Design review of the part built by this model. Coordinates are the model's own, in mm. A direction names the side the tool comes from. Give positions to 0.01 mm unless a question says otherwise; leave off trailing zeros. Order: outer loops, then holes, each group sorted by start corner. A loop starts at its lowest first (then second) coordinate and runs counter-clockwise, first axis right, second up. Notation, with made-up numbers: M -33,61.5 L 1,61.5 A23 ccw 1,71.5 Z; hole C 9,37 d2. An arc over 180 degrees is marked long. Answer as a JSON object with one key per item and string values.
from build123d import *

# Parameters (mm, degrees)
BOSS_EXTRUDE1_DEPTH = 32
SKETCH4_R           = 16
CUT_EXTRUDE3_DEPTH  = 15
SKETCH5_R           = 7
SKETCH5_R_2         = 4
BOSS_EXTRUDE2_DEPTH = 17
SKETCH15_W          = 16
SKETCH15_H          = 32
CUT_EXTRUDE6_DEPTH  = 15
SKETCH16_W          = 32
SKETCH16_H          = 32
BOSS_EXTRUDE6_DEPTH = 20
SKETCH17_R          = 1.75
CUT_EXTRUDE8_DEPTH  = 49
SKETCH18_R          = 1.75
CUT_EXTRUDE9_DEPTH  = 51.695167423
CUT_EXTRUDE10_START = -10
CUT_EXTRUDE10_DEPTH = 5
SKETCH20_R          = 4.25
CUT_EXTRUDE11_DEPTH = 29


with BuildPart() as part:
    # Sketch1 → Boss-Extrude1 (new body)
    with BuildSketch(Plane(origin=(0, 0, 0), x_dir=(0, -1, 0), z_dir=(1, 0, 0))):
        with BuildLine():
            ThreePointArc((-16, 0), (0, 16), (16, 0))
            Line((16, 0), (16, 25))
            Line((16, 25), (-16, 25))
            Line((-16, 25), (-16, 0))
        make_face()
        with BuildLine():
            ThreePointArc((-4.5, 0), (0, 4.5), (4.5, 0))
            Line((4.5, 0), (16, 0))
            ThreePointArc((16, 0), (0, 16), (-16, 0))
            Line((-16, 0), (-4.5, 0))
        make_face()
        with BuildLine():
            Line((16, 0), (4.5, 0))
            ThreePointArc((4.5, 0), (0, -4.5), (-4.5, 0))
            Line((-4.5, 0), (-16, 0))
            ThreePointArc((-16, 0), (0, -16), (16, 0))
        make_face()
        with BuildLine():
            ThreePointArc((-4.5, 0), (0, 4.5), (4.5, 0))
            Line((4.5, 0), (16, 0))
            ThreePointArc((16, 0), (0, 16), (-16, 0))
            Line((-16, 0), (-4.5, 0))
        make_face()
        with BuildLine():
            Line((16, 0), (4.5, 0))
            ThreePointArc((4.5, 0), (0, -4.5), (-4.5, 0))
            Line((-4.5, 0), (-16, 0))
            ThreePointArc((-16, 0), (0, -16), (16, 0))
        make_face()
    extrude(amount=BOSS_EXTRUDE1_DEPTH)

    # Sketch4 → Cut-Extrude3 (cut)
    with BuildSketch(Plane.ZY):
        Circle(SKETCH4_R)
    extrude(amount=-CUT_EXTRUDE3_DEPTH, mode=Mode.SUBTRACT)

    # Sketch5 → Boss-Extrude2 (add)
    with BuildSketch(Plane.ZY.offset(-15)):
        Circle(SKETCH5_R)
        Circle(SKETCH5_R_2, mode=Mode.SUBTRACT)
    extrude(amount=-BOSS_EXTRUDE2_DEPTH)

    # Sketch15 → Cut-Extrude6 (cut)
    with BuildSketch(Plane.ZY):
        with Locations((-8, 0)):
            Rectangle(SKETCH15_W, SKETCH15_H)
    extrude(amount=-CUT_EXTRUDE6_DEPTH, mode=Mode.SUBTRACT)

    # Sketch16 → Boss-Extrude6 (add)
    with BuildSketch(Plane(origin=(0, 0, -25), x_dir=(-1, 0, 0), z_dir=(0, 0, -1))):
        with Locations((-16, 0)):
            Rectangle(SKETCH16_W, SKETCH16_H)
    extrude(amount=BOSS_EXTRUDE6_DEPTH)

    # Sketch17 → Cut-Extrude8 (cut, through all)
    with BuildSketch(Plane.XY.offset(-16)):
        with Locations((4, 0)):
            Circle(SKETCH17_R)
        with Locations((16, 12)):
            Circle(SKETCH17_R)
        with Locations((28, 0)):
            Circle(SKETCH17_R)
        with Locations((16, -12)):
            Circle(SKETCH17_R)
    extrude(amount=-CUT_EXTRUDE8_DEPTH, mode=Mode.SUBTRACT)

    # Sketch18 → Cut-Extrude9 (cut, through all)
    with BuildSketch(Plane.ZY.offset(-15)):
        with Locations((0, 12)):
            Circle(SKETCH18_R)
        with Locations((0, -12)):
            Circle(SKETCH18_R)
        with Locations((12, 0)):
            Circle(SKETCH18_R)
        with Locations(Location((-12, 0, 0), (0, 0, 180))):
            Circle(SKETCH18_R)
    extrude(amount=-CUT_EXTRUDE9_DEPTH, mode=Mode.SUBTRACT)

    # Sketch19 → Cut-Extrude10 (cut)
    with BuildSketch(Plane(origin=(0, 0, -45), x_dir=(-1, 0, 0), z_dir=(0, 0, -1)).offset(CUT_EXTRUDE10_START)):
        Polygon((0, 3), (-5.732050808, 3), (-7.464101615, 0), (-5.732050808, -3), (0, -3), align=None)
        Polygon((-16, -8.535898385), (-19, -10.267949192), (-19, -16), (-13, -16), (-13, -10.267949192), align=None)
        Polygon((-24.535898385, 0), (-26.267949192, 3), (-32, 3), (-32, -3), (-26.267949192, -3), align=None)
        Polygon((-16, 8.535898385), (-13, 10.267949192), (-13, 16), (-19, 16), (-19, 10.267949192), align=None)
    extrude(amount=-CUT_EXTRUDE10_DEPTH, mode=Mode.SUBTRACT)

    # Sketch20 → Cut-Extrude11 (cut)
    with BuildSketch(Plane(origin=(0, 0, -45), x_dir=(-1, 0, 0), z_dir=(0, 0, -1))):
        with Locations((-16, 0)):
            Circle(SKETCH20_R)
    extrude(amount=-CUT_EXTRUDE11_DEPTH, mode=Mode.SUBTRACT)


solid = part.part
(1) Insertion check: pin 1 (4 mm diameter, centred on x = 16, y = 12, fed in from +Z); pin 2 (2 mm diameter, centred on x = 16, y = -12, fed in from -Z); pin 3 (1.5 mm diameter, centred on y = 11.5, z = 7, fed in from -X). Each pin has a flat end and moves straight along its axis. Give the tip position at first contact, or say it passes through.
Checked values:
{"pin 1": "stops at z = 12.49", "pin 2": "stops at z = -16", "pin 3": "stops at x = 15"}
(2) We need section B-B (y = 12). Write out the cut boundary in (x, z).
Checked values:
{"outline": "M 0,-45 L 14.25,-45 L 14.25,-35 L 13,-35 L 13,-30 L 14.25,-30 L 14.25,-16 L 0,-16 Z; M 15,-16 L 17.75,-16 L 17.75,-30 L 19,-30 L 19,-35 L 17.75,-35 L 17.75,-45 L 32,-45 L 32,-1.75 L 15,-1.75 Z; M 15,1.75 L 32,1.75 L 32,10.58 L 15,10.58 Z"}
(3) Tool access review of faces 1 (the flat face through (7, 0, -16)), 2 (the cylindrical face through (26.25, 0.08, -22.9)), 3 (the flat face through (17.5, -9.4, -32.5)), 4 (the flat face through (29, 3, -33)), 5 (the flat face through (6.6, -1.5, -32.5)): name each direction out of +Z, -Z, +X, -X, +Y, -Y from which nothing blocks a thin tool from reaching the whole face with its end or side.
Checked values:
{"face 1": "+Z, -X, +Y, -Y", "face 2": "-Z", "face 3": "-Y", "face 4": "+X", "face 5": "-X"}
(4) We need section D-D (x = 25.5). Write out the cut boundary in (y, z).
Checked values:
{"outline": "M -16,-45 L 16,-45 L 16,0 A16 ccw -16,0 Z; hole C -12,0 d3.5; hole C 0,0 d8; hole C 0,-12 d3.5; hole C 0,12 d3.5; hole M -1.67,-35 L 1.67,-35 L 1.67,-30 L -1.67,-30 Z; hole C 12,0 d3.5"}
(5) We need section A-A (z = -12). Write out the cut boundary in (x, y), plus the area to 4 significant figures.
Checked values:
{"outline": "M 15,-16 L 32,-16 L 32,-1.75 L 15,-1.75 Z; M 15,1.75 L 32,1.75 L 32,16 L 15,16 Z", "area": "484.5 mm^2"}
(6) Draft analysis for pull direction X (two halves, no side actions). For faces 6 (the cylindrical face through (2.25, 0.08, -22.9)), 7 (the flat face through (2, 0, -30)), 8 (the flat face through (0, 0, -27)), state which applies: +X half, -X half, draft (parallel to the pull), parting line (faces both ways), or undercut.
Checked values:
{"face 6": "undercut", "face 7": "draft", "face 8": "-X half"}
(7) To check wall thickness, follow L1, parallel to X at y = 0, z = -34.75; L2, parallel to Y at x = 16, z = -36.25; L3, parallel to Y at x = 24, z = -12. State the ranges of each line that lie inside material, in increasing order. Write a range as from..to.
Checked values:
{"L1": "x = 7.46..11.75, 20.25..24.54", "L2": "y = -16..-13.75, -10.25..-4.25, 4.25..10.25, 13.75..16", "L3": "y = -16..-1.75, 1.75..16"}
(8) We need section C-C (x = 4). Write out the cut boundary in (y, z).
Checked values:
{"outline": "M -16,-45 L -1.75,-45 L -1.75,-35 L -3,-35 L -3,-30 L -1.75,-30 L -1.75,-16 L -16,-16 Z; M 1.75,-45 L 16,-45 L 16,-16 L 1.75,-16 L 1.75,-30 L 3,-30 L 3,-35 L 1.75,-35 Z"}
